The model under review builds one solid part; all positions refer to its coordinate system, in mm. A direction names the side the tool comes from. Coordinates: 2 decimals unless noted, no trailing zeros. Write each loop counter-clockwise with the first axis right and the second up, starting at its lowest first coordinate (ties: lowest second). Pieces come first, ordered by that corner, then holes. Notation, with made-up numbers: (80.5, 14) - (108.5, 14) arc R15 ccw to (108.5, 31) - close; hole circle Ø4 at (44, -18). An arc over 180 degrees is marked (long way). Return JSON: item names as keys, results as strings. Group by question number.
(1) We need section B-B on x = 15. State the section outline as (y, z) points.
(2) We need section A-A on y = -105. State the section outline as (x, z) points (1 decimal).
(3) We need section D-D on z = -1. State the section outline as (x, y) points (1 decimal), then the cut area to 3 significant figures.
(4) Draft analysis for pull direction Y (two halves, no side actions). For faces 1 (the face through (15.462, -98, -6)), 2 (the face through (20.894, -115.267, -4.718)), 3 (the face through (13, -115.888, -3)), state which applies: released by +Y, released by -Y, zero draft, split by the parting line, or undercut.
(5) We need section C-C on z = -6.5. Give the number of separate pieces and of enclosed holes in the cut face, then the cut area to 3 significant figures.
(6) Tool access review of faces 4 (the face through (4.3, -97.45, -4.72)), 5 (the face through (22.225, -106, -4)), 6 (the face through (9.938, -98, -6)), 7 (the face through (13.462, -115, -6)), 8 (the face through (13, -98.711, -4)): name each direction out of +Z, -Z, +X, -X, +Y, -Y from which nothing blocks a thin tool from reaching the whole face with its end or side.
(7) For pin 1 Ø0.5 at (x, y) = (16, -97.5) entering from -Z, flat-tipped, find the tip position at first contact; note if it passes through.
(8) To check wall thickness, follow L1, parallel to Y at x = 12, z = -1.75; L2, parallel to X at y = -113, z = -1 (3 decimals); L3, parallel to Y at x = 16.75, z = -6.5. State the ranges of each line that lie inside material, in increasing order. Write a range as from..to.
```python
from build123d import *

# Parameters (mm, degrees)
SKETCH1_W                 = 19.05
SKETCH1_H                 = 19.05
SKETCH1_W_2               = 15.3035
SKETCH1_H_2               = 15.3035
BOSS_EXTRUDE1_DEPTH       = 7.9375
SKETCH2_W                 = 1.524
SKETCH2_H                 = 1.87325
CUT_EXTRUDE_THIN1_DEPTH   = 4.699
FILLET2_R                 = 0.508
CHAMFER1_SIZE             = 0.762
F_0_80_TAPPED_HOLE1_D     = 1.19126
F_0_80_TAPPED_HOLE1_DEPTH = 6.35
F_0_80_TAPPED_HOLE1_TIP   = 0.357890611


with BuildPart() as part:
    # Sketch1 → Boss-Extrude1 (new body)
    with BuildSketch(Plane.XY):
        with Locations((12.7, -106.3625)):
            Rectangle(SKETCH1_W, SKETCH1_H)
        with Locations((12.7, -106.3625)):
            Rectangle(SKETCH1_W_2, SKETCH1_H_2, mode=Mode.SUBTRACT)
    extrude(amount=-BOSS_EXTRUDE1_DEPTH)

    # Sketch2 → Cut-Extrude-Thin1 (cut)
    with BuildSketch(Plane(origin=(0, 0, -7.9375), x_dir=(-1, 0, 0), z_dir=(0, 0, -1))):
        with Locations((-12.7, -114.950875)):
            Rectangle(SKETCH2_W, SKETCH2_H)
        with Locations((-9.17575, -97.774125)):
            Rectangle(SKETCH2_W, SKETCH2_H)
        with Locations((-16.22425, -97.774125)):
            Rectangle(SKETCH2_W, SKETCH2_H)
    extrude(amount=-CUT_EXTRUDE_THIN1_DEPTH, mode=Mode.SUBTRACT)

    # Fillet2
    fillet2_edges = [part.edges().sort_by_distance(p)[0] for p in [
        (12.7, -96.8375, 0),
        (22.225, -106.3625, 0),
        (12.7, -115.8875, 0),
        (3.175, -106.3625, 0),
        (3.175, -96.8375, -3.96875),
        (22.225, -96.8375, -3.96875),
        (22.225, -115.8875, -3.96875),
        (3.175, -115.8875, -3.96875),
    ]]
    fillet(fillet2_edges, radius=FILLET2_R)

    # Chamfer1
    chamfer1_edges = [part.edges().sort_by_distance(p)[0] for p in [
        (5.04825, -114.01425, -3.96875),
        (5.04825, -98.71075, -3.96875),
        (20.35175, -98.71075, -3.96875),
        (20.35175, -114.01425, -3.96875),
    ]]
    chamfer(chamfer1_edges, length=CHAMFER1_SIZE)

    # #0-80 Tapped Hole1
    with Locations(Plane(origin=(0, 0, -7.9375), x_dir=(-1, 0, 0), z_dir=(0, 0, -1))):
        with Locations((-4.376519878, -98.039019878), (-21.023480122, -114.685980122)):
            Hole(F_0_80_TAPPED_HOLE1_D / 2, depth=F_0_80_TAPPED_HOLE1_DEPTH)
            with Locations((0, 0, -(F_0_80_TAPPED_HOLE1_DEPTH + F_0_80_TAPPED_HOLE1_TIP / 2))):  # 118° drill point
                Cone(0, F_0_80_TAPPED_HOLE1_D / 2, F_0_80_TAPPED_HOLE1_TIP, mode=Mode.SUBTRACT)


solid = part.part
```
Ans:
{
 "1": {"outline": "(-115.89, -7.94) - (-114.01, -7.94) - (-114.01, 0) - (-115.38, 0) arc R0.51 ccw to (-115.89, -0.51) - close; (-98.71, -7.94) - (-96.84, -7.94) - (-96.84, -0.51) arc R0.51 ccw to (-97.35, 0) - (-98.71, 0) - close"},
 "2": {"outline": "(3.2, -7.9) - (5, -7.9) - (5, 0) - (3.7, 0) arc R0.5 ccw to (3.2, -0.5) - close; (20.4, -7.9) - (22.2, -7.9) - (22.2, -0.5) arc R0.5 ccw to (21.7, 0) - (20.4, 0) - close"},
 "3": {"outline": "(3.2, -115.4) arc R0.5 ccw to (3.7, -115.9) - (21.7, -115.9) arc R0.5 ccw to (22.2, -115.4) - (22.2, -97.3) arc R0.5 ccw to (21.7, -96.8) - (3.7, -96.8) arc R0.5 ccw to (3.2, -97.3) - close; hole (5, -113.3) - (5.8, -114) - (19.6, -114) - (20.4, -113.3) - (20.4, -99.5) - (19.6, -98.7) - (5.8, -98.7) - (5, -99.5) - close", "area": "130 mm²"},
 "4": {"face 1": "zero draft", "face 2": "undercut", "face 3": "released by -Y"},
 "5": {"separate pieces": "3", "enclosed holes": "2", "area": "119 mm²"},
 "6": {"face 4": "-Z", "face 5": "+Z, -Z, +X, +Y, -Y", "face 6": "-Z, +Y", "face 7": "-Z, -Y", "face 8": "+Z, -Z"},
 "7": {"pin 1": "z = -3.24"},
 "8": {"L1": "-115.89..-114.01, -98.71..-96.84", "L2": "3.175..5.048, 20.352..22.225", "L3": "-115.89..-114.01"}
}
